Read the model definition and answer for the solid it produces. Units are mm, in the model's axes. Coordinates: 2 decimals unless noted, no trailing zeros. Loops run counter-clockwise (first coordinate to the right, second up) from the corner with the lowest first, then second, coordinate; pieces in that order, holes last.
from build123d import *

# Parameters (mm, degrees)
F0_W     = 79.1259
F0_H     = 5.074583
F0_W_2   = 84.01253
F0_H_2   = 4.510738
F0_W_3   = 85.328166
F0_H_3   = 5.262531
F0_W_4   = 88.523269
F0_H_4   = 5.826373
F0_W_5   = 89.275062
F0_H_5   = 6.578165
F0_W_6   = 85.328165
F0_H_6   = 6.766111
F1_DEPTH = 0.5


with BuildPart() as f1:
    # F0 (on Front) → F1 (new body)
    with BuildSketch(Plane.XZ):
        Polygon((62.676273, 71.898557), (-58.361914, 71.898557), (-58.361914, 47.371406), (-8.367877, 47.371406), (-8.367877, 42.390797), (-58.361914, 42.390797), (-58.361914, 22.844255), (-7.616087, 22.844255), (-7.616087, 18.145567), (-58.361914, 18.145567), (-58.361914, -2.34071), (-10.247352, -2.34071), (-10.247352, -7.415293), (-58.361914, -7.415293), (-58.361914, -22.826988), (-7.428139, -22.826988), (-7.428139, -26.585938), (-58.361914, -26.585938), (-58.361914, -43.313265), (-4.608927, -43.313265), (-4.608927, -46.69632), (-58.361914, -46.69632), (-58.361914, -63.2357), (-4.796875, -63.2357), (-4.796875, -66.994652), (-58.361914, -66.994652), (-58.361914, -72.821021), (62.676273, -72.821021), (62.676273, -66.994652), (4.224605, -66.994652), (4.224605, -63.2357), (62.676273, -63.2357), (62.676273, -46.69632), (5.540238, -46.69632), (5.540238, -43.313265), (62.676273, -43.313265), (62.676273, -26.585938), (6.10408, -26.585938), (6.10408, -22.826988), (62.676273, -22.826988), (62.676273, -7.415293), (9.675083, -7.415293), (9.675083, -2.34071), (62.676273, -2.34071), (62.676273, 18.145567), (7.983554, 18.145567), (7.983554, 22.844255), (62.676273, 22.844255), (62.676273, 42.390797), (11.178663, 42.390797), (11.178663, 47.371406), (62.676273, 47.371406), align=None)
        with Locations((3.754737, -56.563564)):
            Rectangle(F0_W, F0_H, mode=Mode.SUBTRACT)
        with Locations((6.573949, -35.983313)):
            Rectangle(F0_W_2, F0_H_2, mode=Mode.SUBTRACT)
        with Locations((6.10408, -15.309088)):
            Rectangle(F0_W_3, F0_H_3, mode=Mode.SUBTRACT)
        with Locations((5.822159, 7.338586)):
            Rectangle(F0_W_4, F0_H_4, mode=Mode.SUBTRACT)
        with Locations((5.446263, 31.395866)):
            Rectangle(F0_W_5, F0_H_5, mode=Mode.SUBTRACT)
        with Locations((5.35229, 55.73507)):
            Rectangle(F0_W_6, F0_H_6, mode=Mode.SUBTRACT)
    extrude(amount=F1_DEPTH)


solid = f1.part
Q1. Straight lines are drawn through the part: probe 1 along X at (y, z) = (-0.35, -14); probe 2 along X at (y, z) = (-0.4, -46); probe 3 along X at (y, z) = (-0.3, -23). For each, find the intervals that lie inside material, in ascending order.
Findings below:
probe 1: x = -58.36 to -36.56, 48.77 to 62.68
probe 2: x = -4.61 to 5.54
probe 3: x = -7.43 to 6.1
Q2. A cutting plane is placed at B-B (z = 8.5). Give the vertices of the cut face in (x, y).
Findings below:
outline: (-58.36, -0.5) - (-38.44, -0.5) - (-38.44, 0) - (-58.36, 0) - close; (50.08, -0.5) - (62.68, -0.5) - (62.68, 0) - (50.08, 0) - close
Q3. A cutting plane is placed at C-C (y = -0.4). Count the separate pieces of the cut face and the enclosed holes in it, then the cut area to 3 significant figures.
Findings below:
separate pieces: 1
enclosed holes: 6
area: 11,900 mm2
Q4. A cutting plane is placed at A-A (x = -42). Give the vertices of the cut face in (y, z).
Findings below:
outline: (-0.5, -72.82) - (0, -72.82) - (0, -66.99) - (-0.5, -66.99) - close; (-0.5, -63.24) - (0, -63.24) - (0, -46.7) - (-0.5, -46.7) - close; (-0.5, -43.31) - (0, -43.31) - (0, -26.59) - (-0.5, -26.59) - close; (-0.5, -22.83) - (0, -22.83) - (0, -7.42) - (-0.5, -7.42) - close; (-0.5, -2.34) - (0, -2.34) - (0, 18.15) - (-0.5, 18.15) - close; (-0.5, 22.84) - (0, 22.84) - (0, 42.39) - (-0.5, 42.39) - close; (-0.5, 47.37) - (0, 47.37) - (0, 71.9) - (-0.5, 71.9) - close
